The listing builds one solid part. Answer for the finished solid, in the listing's coordinates (mm). A direction names the side the tool comes from. Give positions to 0.01 mm unless a question says otherwise; leave off trailing zeros. Order: outer loops, then holes, each group sorted by start corner. A loop starts at its lowest first (then second) coordinate and runs counter-clockwise, first axis right, second up.
```python
from build123d import *

# Parameters (mm, degrees)
CROQUIS1_R              = 7.000000002
SALIENTE_EXTRUIR1_DEPTH = 3
CROQUIS2_W              = 33.4
CROQUIS2_H              = 3
SALIENTE_EXTRUIR2_DEPTH = 41.4
CROQUIS3_R              = 7.000000002
SALIENTE_EXTRUIR3_DEPTH = 3


with BuildPart() as part:
    # Croquis1 → Saliente-Extruir1 (new body)
    with BuildSketch(Plane(origin=(0, 0, 0), x_dir=(0, 0, -1), z_dir=(1, 0, 0))):
        with BuildLine():
            Line((16.7, 25), (16.7, 0))
            Line((16.7, 0), (-16.7, 0))
            Line((-16.7, 0), (-16.7, 25))
            ThreePointArc((-16.7, 25), (0, 41.7), (16.7, 25))
        make_face()
        with Locations((0, 25)):
            Circle(CROQUIS1_R, mode=Mode.SUBTRACT)
    extrude(amount=SALIENTE_EXTRUIR1_DEPTH)

    # Croquis2 → Saliente-Extruir2 (add)
    with BuildSketch(Plane(origin=(3, 0, 0), x_dir=(0, 0, -1), z_dir=(1, 0, 0))):
        with Locations((0, -1.5)):
            Rectangle(CROQUIS2_W, CROQUIS2_H)
    extrude(amount=-SALIENTE_EXTRUIR2_DEPTH)

    # Croquis3 → Saliente-Extruir3 (add)
    with BuildSketch(Plane.ZY.offset(38.4)):
        with BuildLine():
            Line((16.7, 0), (16.7, 25))
            ThreePointArc((16.7, 25), (0, 41.7), (-16.7, 25))
            Line((-16.7, 25), (-16.7, 0))
            Line((-16.7, 0), (16.7, 0))
        make_face()
        with Locations((0, 25)):
            Circle(CROQUIS3_R, mode=Mode.SUBTRACT)
    extrude(amount=-SALIENTE_EXTRUIR3_DEPTH)


solid = part.part
```
1) For a pull along Y with two mould halves and no side action, classify faces 1 (the cylindrical face through (-36.921, 18.166, -1.517)), 2 (the flat face through (0, 17, 0)), 3 (the cylindrical face through (-36.921, 41.696, 0.367)), 4 (the cylindrical face through (1.479, 18.166, 1.517)) as +Y half, -Y half, draft (parallel to the pull), parting line (faces both ways), or undercut.
Geometry says:
face 1: undercut
face 2: draft
face 3: +Y half
face 4: undercut
2) Straight lines are drawn through the part: probe 1 along X at (y, z) = (35, -5); probe 2 along Y at (x, z) = (1.1, 0); probe 3 along Y at (x, z) = (-16, -3.5). For each, find the intervals that lie inside material, in ascending order.
Geometry says:
probe 1: x = -38.4 to -35.4, 0 to 3
probe 2: y = -3 to 18, 32 to 41.7
probe 3: y = -3 to 0
3) Find section B-B (y = 4.5). Write down the section's boundary in (x, z), then the cut area to 3 significant figures.
Geometry says:
outline: (-38.4, -16.7) - (-35.4, -16.7) - (-35.4, 16.7) - (-38.4, 16.7) - close; (0, -16.7) - (3, -16.7) - (3, 16.7) - (0, 16.7) - close
area: 200 mm2
4) Find section A-A (z = 0). Write down the section's boundary in (x, y).
Geometry says:
outline: (-38.4, -3) - (3, -3) - (3, 18) - (0, 18) - (0, 0) - (-35.4, 0) - (-35.4, 18) - (-38.4, 18) - close; (-38.4, 32) - (-35.4, 32) - (-35.4, 41.7) - (-38.4, 41.7) - close; (0, 32) - (3, 32) - (3, 41.7) - (0, 41.7) - close
5) Given P1, Ø8, axis at x = -12, z = -10, coming from the +Y side; P2, Ø5, axis at x = -33.5, z = -5.5, coming from the +Y side, each flat-ended and moving along its own axis, determine where each tip first touches the part or whether it passes through.
Geometry says:
P1: stops at y = 0
P2: stops at y = 41.24
6) A tool of negligible diameter and unlimited length cuts with its end or side. For faces 5 (the flat face through (-35.4, 17, 0)), 6 (the flat face through (-17, -3, 0)), from which of +Z, -Z, +X, -X, +Y, -Y can it reach the whole face along a straight path? Write none if from no direction.
Geometry says:
face 5: +Z, -Z, +Y
face 6: +Z, -Z, +X, -X, -Y
7) Find section C-C (y = 21). Write down the section's boundary in (x, z), then the cut area to 3 significant figures.
Geometry says:
outline: (-38.4, -16.7) - (-35.4, -16.7) - (-35.4, -5.74) - (-38.4, -5.74) - close; (-38.4, 5.74) - (-35.4, 5.74) - (-35.4, 16.7) - (-38.4, 16.7) - close; (0, -16.7) - (3, -16.7) - (3, -5.74) - (0, -5.74) - close; (0, 5.74) - (3, 5.74) - (3, 16.7) - (0, 16.7) - close
area: 131 mm2
8) Find section D-D (x = -4.5). Write down the section's boundary in (y, z).
Geometry says:
outline: (-3, -16.7) - (0, -16.7) - (0, 16.7) - (-3, 16.7) - close
